Check sheet for the drawn part. Datum: minimum x, y, z corner. Units: mm. A direction names the side the tool comes from. Give positions to 0.01 mm unless a question says otherwise; leave off trailing zeros. Order: outer loops, then holes, each group sorted by start corner. A loop starts at its lowest first (then second) coordinate and runs counter-clockwise, first axis right, second up.
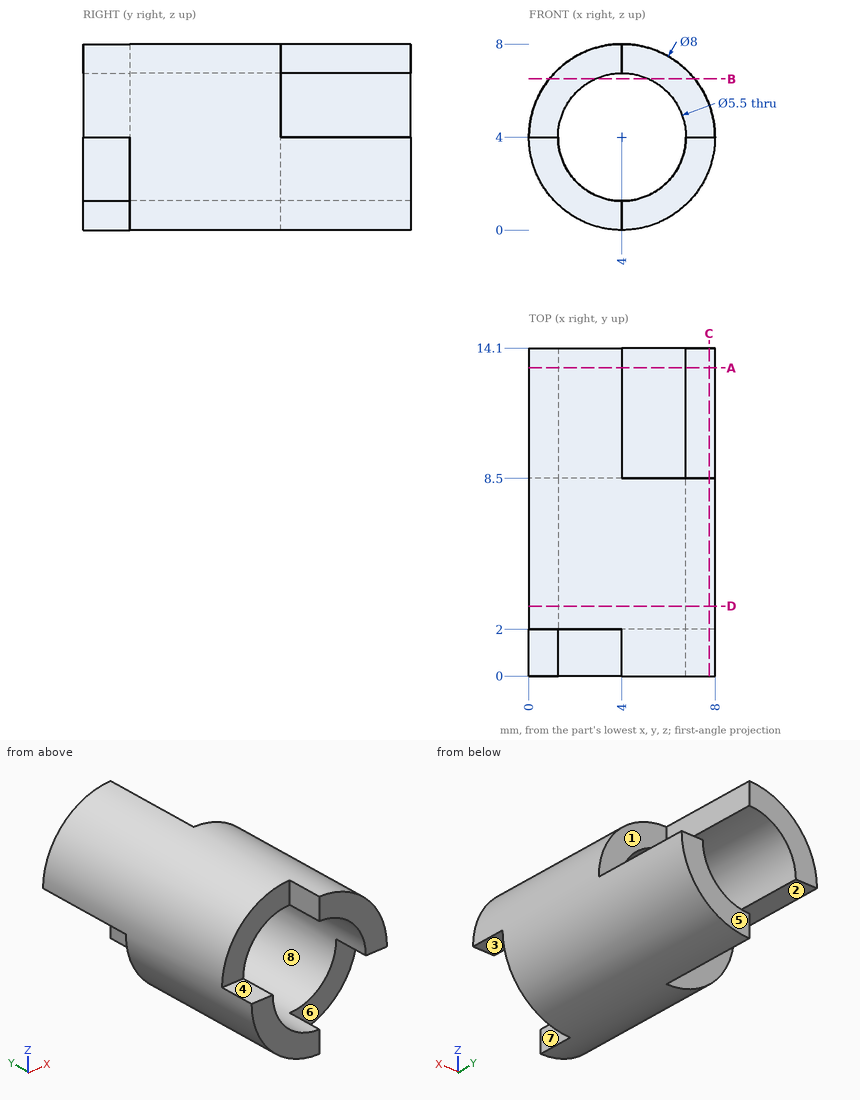
Q1. Sectioned sample at C-C, the plane x = 7.75. Record the cut outline in (y, z), plus the area to 3 significant figures.
Q2. Sectioned sample at A-A, the plane y = 13.25. Record the cut outline in (x, z), plus the area to 3 significant figures.
Q3. Tool access check on the marked faces 1, 2, 3, 4 and 5. Record the directions out of +Z, -Z, +X, -X, +Y, -Y that give a thin tool (end or side, any length) a straight path to the whole face; none if there is none.
Q4. Draft check along X on the marked faces 6, 7 and 8. Enter one of: pulls with the +X half, pulls with the -X half, needs draft (parallel to the pull), parting line crosses it, or undercut.
Q5. Go/stop test with flat-tipped pins: P1, Ø1.4, axis at y = 10.5, z = 0.5, coming from the -X side; P2, Ø2, axis at y = 5, z = 7, coming from the -X side; P3, Ø0.6, axis at x = 7, y = 1, coming from the -Z side; P4, Ø2, axis at x = 4.5, z = 5, coming from the -Y side. Record where each tip stops, or that it passes through.
Q6. Sectioned sample at B-B, the plane z = 6.5. Record the cut outline in (x, y), plus the area to 3 significant figures.
Q7. Sectioned sample at D-D, the plane y = 3. Record the cut outline in (x, z), plus the area to 3 significant figures.
Q8. Material ranges on line 1 (X direction, y = 5.5, z = 4); line 2 (Y direction, x = 2.25, z = 7.5); line 3 (X direction, y = 6, z = 6), recorded low to high.
Filled in:
1. outline: (0, 4) - (2, 4) - (2, 2.61) - (14.1, 2.61) - (14.1, 4) - (8.5, 4) - (8.5, 5.39) - (0, 5.39) - close
1. area: 28.7 mm2
2. outline: (0, 4) - (1.25, 4) arc R2.75 cw to (4, 6.75) - (4, 8) arc R4 ccw to start; (4, 0) arc R4 ccw to (8, 4) - (6.75, 4) arc R2.75 cw to (4, 1.25) - close
2. area: 13.3 mm2
3. face 1: +Z, +X, +Y
3. face 2: -Z, -X, +Y
3. face 3: -Z, +X, -Y
3. face 4: +Z, -X, -Y
3. face 5: +Z, -Z, +X, -X, +Y
4. face 6: needs draft
4. face 7: pulls with the +X half
4. face 8: undercut
5. P1: stops at x = 4
5. P2: stops at x = 0.54
5. P3: stops at z = 4
5. P4: passes through
6. outline: (0.88, 2) - (2.85, 2) - (2.85, 14.1) - (0.88, 14.1) - close; (5.15, 0) - (7.12, 0) - (7.12, 8.5) - (5.15, 8.5) - close
6. area: 40.7 mm2
7. outline: circle Ø8 at (4, 4); hole circle Ø5.5 at (4, 4)
7. area: 26.5 mm2
8. line 1: x = 0 to 1.25, 6.75 to 8
8. line 2: y = 2 to 14.1
8. line 3: x = 0.54 to 2.11, 5.89 to 7.46
